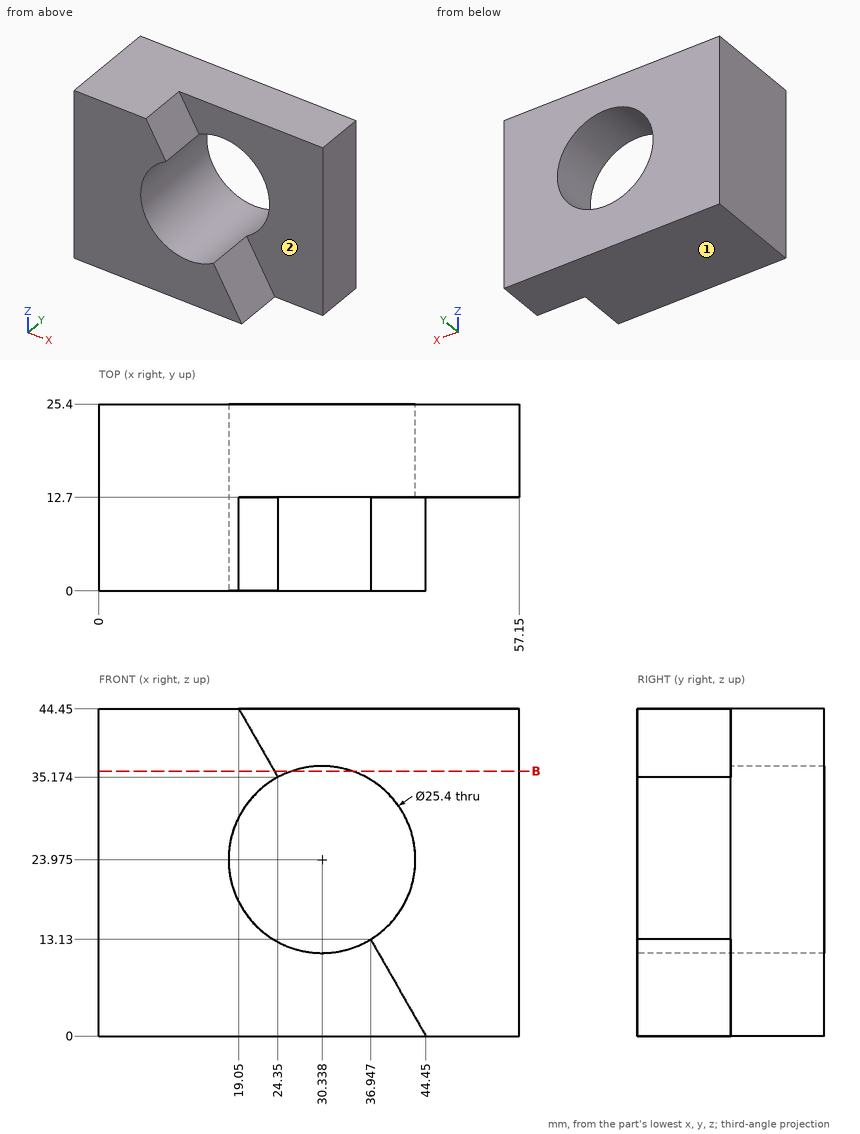
Source: three-view drawing plus pictorial views. Frame: mm from the lowest corner of the part. A direction names the side the tool comes from. Give positions to 0.01 mm unless a question says otherwise; leave off trailing zeros. Loops run counter-clockwise (first coordinate to the right, second up) from the corner with the lowest first, then second, coordinate; pieces in that order, holes last. Notation, with made-up numbers: (-9.5, 38) -> (3.5, 38) arc R26 cw to (3.5, 66) -> close; hole circle Ø4 at (50, 42.25). An arc over 180 degrees is marked (long way). Use a Markdown table: item, result. Add a question column.
(1) Ray query, line 1 (Z direction, x = 23, y = 21.75); line 2 (Z direction, x = 28.5, y = 19); line 3 (Y direction, x = 47, z = 34.5). Return the intervals inside material, ascending.
(2) Access query for the marked faces 1 and 2. Directions: +Z, -Z, +X, -X, +Y, -Y. A direction counts if a zero-diameter tool reaches every point of the face in a straight line with its end or side. Return the directions, or none.
(3) First-contact query: pin 1 Ø1 at (x, y) = (37.5, 2.5) entering from +Z (1 decimal); pin 2 Ø12 at (x, z) = (48.5, 15) entering from -Y. Flat tips, straight axial feed; report the tip coordinate or a pass-through.
(4) Section query B-B (z = 36). Output: boundary loops of the cut face in (x, y).
Checked values:
| question | item | result |
|---|---|---|
| 1 | line 1 | 0 to 13.61, 34.34 to 44.45 |
| 1 | line 2 | 0 to 11.41, 36.54 to 44.45 |
| 1 | line 3 | 12.7 to 25.4 |
| 2 | face 1 | -Z, +X, -X, +Y, -Y |
| 2 | face 2 | +Z, +X, -Y |
| 3 | pin 1 | z = 13 |
| 3 | pin 2 | y = 12.7 |
| 4 | outline | (0, 0) -> (23.88, 0) -> (23.88, 12.7) -> (26.25, 12.7) -> (26.25, 25.4) -> (0, 25.4) -> close; (34.42, 12.7) -> (57.15, 12.7) -> (57.15, 25.4) -> (34.42, 25.4) -> close |
